Build history of the part. All positions in model axes, mm. A direction names the side the tool comes from. Coordinates: 2 decimals unless noted, no trailing zeros. Loops run counter-clockwise (first coordinate to the right, second up) from the corner with the lowest first, then second, coordinate; pieces in that order, holes last.
(1) Tool access for faces 4 (the face through (-8.788, 4.9, 11.5)), 5 (the face through (10, 5, 14.795)), 6 (the face through (0, 5, -5.414)), 7 (the face through (5.482, 5, 0)): list every direction of +Z, -Z, +X, -X, +Y, -Y with a clear straight run to the whole face (end or side of a thin tool).
(2) Slice it at A-A (z = 0). Give the cut face in (x, y).
(3) Slice it at B-B (x = 0). Give the cut face in (y, z), and give its area (3 significant figures).
(4) Flat gauge pins, fed straight in: P1, Ø1, axis at x = 3, y = 2.5, coming from the -Z side; P2, Ø5.5, axis at y = 6, z = -0.5, coming from the -X side; P3, Ø5, axis at x = 9.5, y = 4, coming from the +Z side (3 decimals). Where does each tip first touch, or does it go through?
(5) Slice it at C-C (z = -8). Give the cut face in (x, y).
(6) Two-plate mould, pull along X, no slides. Class faces 1 (the face through (-15, 5, -9)), 2 (the face through (-8.066, 4.93, -6.612)), 3 (the face through (-14, 5, 4.218)): pulls with the +X half, pulls with the -X half, needs draft (parallel to the pull), parting line crosses it, or undercut.
(7) Wall check: L1, parallel to X at y = 6, z = 0; L2, parallel to Z at x = 0, y = 6.75; L3, parallel to X at y = 0.5, z = -12. Give the ranges that are in metal, low to high.
Autodesk Inventor part; units mm, degrees
ref_plane "YZ Plane" through (0, 0, 0) normal (1, 0, 0) x (0, 1, 0)
ref_plane "XZ Plane" through (0, 0, 0) normal (0, 1, 0) x (-1, 0, 0)
ref_plane "XY Plane" through (0, 0, 0) normal (0, 0, 1) x (1, 0, 0)
sketch "Sketch1" plane through (0, 0, 0) normal (0, 1, 0) x (-1, 0, 0)
  line L0 (0, -21.0136) -> (0, 21.0817)
  line L1 (-21, 0) -> (21, 0)
  line L2 (21, 0) -> (-21, 0)
  line L3 (0, -21.0136) -> (0, 21.0817)
  line L4 (3.6865, 5.4825) -> (-4.0965, 5.4825)
  line L5 (-5.4825, 3.7546) -> (-5.4825, -4.0284)
  line L6 (-4.0967, -5.4144) -> (3.6863, -5.4144)
  line L7 (5.4825, -4.0284) -> (5.4825, 3.7546)
  line L8 (-5.4825, 5.4825) -> (5.4825, -5.4825) construction
  line L9 (15, 15.0681) -> (15, 4.2181)
  line L10 (15, 4.2181) -> (12.75, 4.2181)
  line L11 (15, 15.0681) -> (4.15, 15.0681)
  line L12 (4.15, 15.0681) -> (4.15, 12.8181)
  line L13 (-15, 14.795) -> (-4.15, 14.795)
  line L14 (-4.15, 14.795) -> (-4.15, 12.75)
  line L15 (-15, 12.75) -> (-15, 14.795)
  line L16 (-15, 14.795) -> (-12.75, 14.795)
  line L17 (-12.75, 3.945) -> (-15, 3.945)
  line L18 (-15, 3.945) -> (-15, 14.795)
  line L19 (-15, -14.9319) -> (-12.75, -14.9319)
  line L20 (-12.75, -4.0819) -> (-15, -4.0819)
  line L21 (-15, -4.0819) -> (-15, -14.9319)
  line L22 (-15, -14.9319) -> (-4.1502, -14.9319)
  line L23 (-4.1502, -14.9319) -> (-4.1502, -12.6819)
  line L24 (-15, -12.7481) -> (-15, -14.9319)
  line L25 (15, -14.9319) -> (12.75, -14.9319)
  line L26 (12.75, -4.0819) -> (15, -4.0819)
  line L27 (15, -4.0819) -> (15, -14.9319)
  line L28 (15, -14.9319) -> (4.1502, -14.9319)
  line L29 (4.1502, -14.9319) -> (4.1502, -12.6819)
  line L30 (15, -12.7481) -> (15, -14.9319)
  circle A0 centre (0, 0) radius 3.1425
  line L31 (8.9925, -14.9319) -> (4.1502, -14.9319)
  line L32 (-4.1502, -14.9319) -> (-8.9925, -14.9319)
  line L33 (15, -14.9319) -> (4.1502, -14.9319)
  line L34 (-4.1502, -14.9319) -> (-15, -14.9319)
  line L35 (15, -8.9925) -> (15, -4.0819)
  line L36 (15, 4.2181) -> (15, 9.0606)
  line L37 (15, 15.0681) -> (15, 4.2181)
  line L38 (15, -4.0819) -> (15, -14.9319)
  line L39 (-8.9925, 14.795) -> (-4.15, 14.795)
  line L40 (4.15, 15.0681) -> (8.9925, 15.0681)
  line L41 (-15, 14.795) -> (-4.15, 14.795)
  line L42 (4.15, 15.0681) -> (15, 15.0681)
  line L43 (-15, 8.9925) -> (-15, 3.945)
  line L44 (-15, -4.0819) -> (-15, -8.9925)
  line L45 (-15, -14.9319) -> (-15, -4.0819)
  line L46 (-15, 3.945) -> (-15, 14.795)
  line L47 (-4.1502, -12.6819) -> (-9.1977, -12.6819)
  line L48 (-12.75, -9.1294) -> (-12.75, -4.0819)
  line L49 (-12.75, -9.1294) -> (-10.5835, -9.1294)
  line L50 (-9.1977, -12.6819) -> (-9.1977, -10.5154)
  line L51 (-9.1975, 10.5835) -> (-9.1975, 12.75)
  line L52 (4.15, 12.8181) -> (8.7875, 12.8181)
  line L53 (12.75, 4.2181) -> (12.75, 8.8556)
  line L54 (12.75, 8.8556) -> (10.5835, 8.8556)
  line L55 (8.7875, 12.8181) -> (8.7875, 10.5835)
  line L56 (4.1502, -12.6819) -> (8.7873, -12.6819)
  line L57 (14.341, -12.7481) -> (15, -12.7481)
  line L58 (12.75, -14.9319) -> (12.75, -14.2729)
  line L59 (12.75, -9.1294) -> (12.75, -4.0819)
  line L60 (10.5835, -9.1294) -> (12.75, -9.1294)
  line L61 (8.7873, -10.5154) -> (8.7873, -12.6819)
  line L62 (5.4825, 5.4825) -> (-0.7955, -0.7955) construction
  line L63 (-2.2221, -2.2221) -> (-5.4825, -5.4825) construction
  line L64 (-12.75, 14.795) -> (-12.75, 14.136)
  line L65 (-12.75, 8.8556) -> (-12.75, 3.945)
  line L66 (-4.15, 12.75) -> (-9.1975, 12.75)
  line L67 (-14.341, 12.75) -> (-15, 12.75)
  line L68 (-10.5835, 8.8556) -> (-12.75, 8.8556)
  line L69 (-5.4825, 3.7546) -> (-10.5835, 8.8556)
  line L70 (-4.0965, 5.4825) -> (-9.1975, 10.5835)
  line L71 (8.7875, 10.5835) -> (3.6865, 5.4825)
  line L72 (10.5835, 8.8556) -> (5.4825, 3.7546)
  line L73 (10.5835, -9.1294) -> (5.4825, -4.0284)
  line L74 (8.7873, -10.5154) -> (3.6863, -5.4144)
  line L75 (-4.0967, -5.4144) -> (-9.1977, -10.5154)
  line L76 (-5.4825, -4.0284) -> (-10.5835, -9.1294)
  line L77 (15, 15) -> (-15, -15) construction
  line L78 (-15, 15) -> (15, -15) construction
  point P0 (-15, 0)
  dimension "d26" = 6.285
  dimension "d0" = 30
  dimension "d1" = 30
  dimension "d2" = 10.965
  dimension "d3" = 10.965
  dimension "d4" = 30
  dimension "d5" = 17.985
  dimension "d6" = 17.985
  dimension "d11" = 10.85
  dimension "d12" = 2.25
  dimension "d13" = 10.85
  dimension "d14" = 2.25
  dimension "d15" = 10.85
  dimension "d16" = 2.25
  dimension "d17" = 10.85
  dimension "d18" = 2.25
  dimension "d19" = 10.85
  dimension "d20" = 10.85
  dimension "d21" = 2.25
  dimension "d22" = 2.25
  dimension "d23" = 10.85
  dimension "d24" = 10.85
  dimension "d25" = 2.25
  dimension "d31" = 30
  dimension "d32" = 30
extrude "Extrusion1" add sketch "Sketch1" along normal blind 10 contours L6 L75 L50 L47 L23 L22 L19 L21 L20 L48 L49 L76 L5 L1 A0 L0 | L0 A0 L1 L7 L73 L60 L59 L26 L27 L25 L28 L29 L56 L61 L74 L6 | L1 L5 L69 L68 L65 L17 L18 L15 L13 L14 L66 L51 L70 L4 L0 A0 | A0 L0 L4 L71 L55 L52 L12 L11 L9 L10 L53 L54 L72 L7 L1
fillet "Fillet1" radius 0.5 20 edges at (15, 5, 14.795) (4.15, 5, 14.795) (-4.15, 5, 15.0681) (-4.15, 5, 12.8181) (15, 5, 3.945) (12.75, 5, 3.945) (15, 5, -4.0819) (12.75, 5, -4.0819) (15, 5, -14.9319) (4.1502, 5, -12.6819) (-4.1502, 5, -14.9319) (-4.1502, 5, -12.6819) (4.1502, 5, -14.9319) (-15, 5, -14.9319) (-12.75, 5, -4.0819) (-15, 5, -4.0819) (-12.75, 5, 4.2181) (-15, 5, 4.2181) (-15, 5, 15.0681) (4.15, 5, 12.75)
fillet "Fillet2" radius 0.75 24 edges at (-10.5835, 5, 8.8556) (-5.4825, 5, 3.7546) (-12.75, 5, -9.1294) (-10.5835, 5, -9.1294) (-8.7873, 5, -12.6819) (5.4825, 5, -4.0284) (10.5835, 5, -9.1294) (-3.6865, 5, 5.4825) (-8.7875, 5, 10.5835) (5.4825, 5, 3.7546) (10.5835, 5, 8.8556) (12.75, 5, 8.8556) (12.75, 5, -9.1294) (4.0965, 5, 5.4825) (9.1975, 5, 10.5835) (9.1975, 5, 12.75) (-8.7875, 5, 12.8181) (-12.75, 5, 8.8556) (4.0967, 5, -5.4144) (9.1977, 5, -10.5154) (9.1977, 5, -12.6819) (-8.7873, 5, -10.5154) (-3.6863, 5, -5.4144) (-5.4825, 5, -4.0284)
properties part number "Profile_iPart"
Response values:
1. face 4: +Y, -Y
1. face 5: +Z, +X, +Y, -Y
1. face 6: -Z, +Y, -Y
1. face 7: +X, +Y, -Y
2. outline: (-5.48, 0) - (-3.14, 0) - (-3.14, 10) - (-5.48, 10) - close; (3.14, 0) - (5.48, 0) - (5.48, 10) - (3.14, 10) - close
3. outline: (0, -5.41) - (10, -5.41) - (10, -3.14) - (0, -3.14) - close; (0, 3.14) - (10, 3.14) - (10, 5.48) - (0, 5.48) - close
3. area: 46.1 mm2
4. P1: stops at z = -5.41
4. P2: stops at x = -5.48
4. P3: stops at z = 14.795
5. outline: (-15, 0) - (-12.75, 0) - (-12.75, 10) - (-15, 10) - close; (-9.45, 0) - (-6.27, 0) - (-6.27, 10) - (-9.45, 10) - close; (6.68, 0) - (9.45, 0) - (9.45, 10) - (6.68, 10) - close; (12.75, 0) - (15, 0) - (15, 10) - (12.75, 10) - close
6. face 1: pulls with the -X half
6. face 2: undercut
6. face 3: needs draft
7. L1: x = -5.48 to -3.14, 3.14 to 5.48
7. L2: z = -5.41 to -3.14, 3.14 to 5.48
7. L3: x = -15 to -8.78, 9.19 to 15
